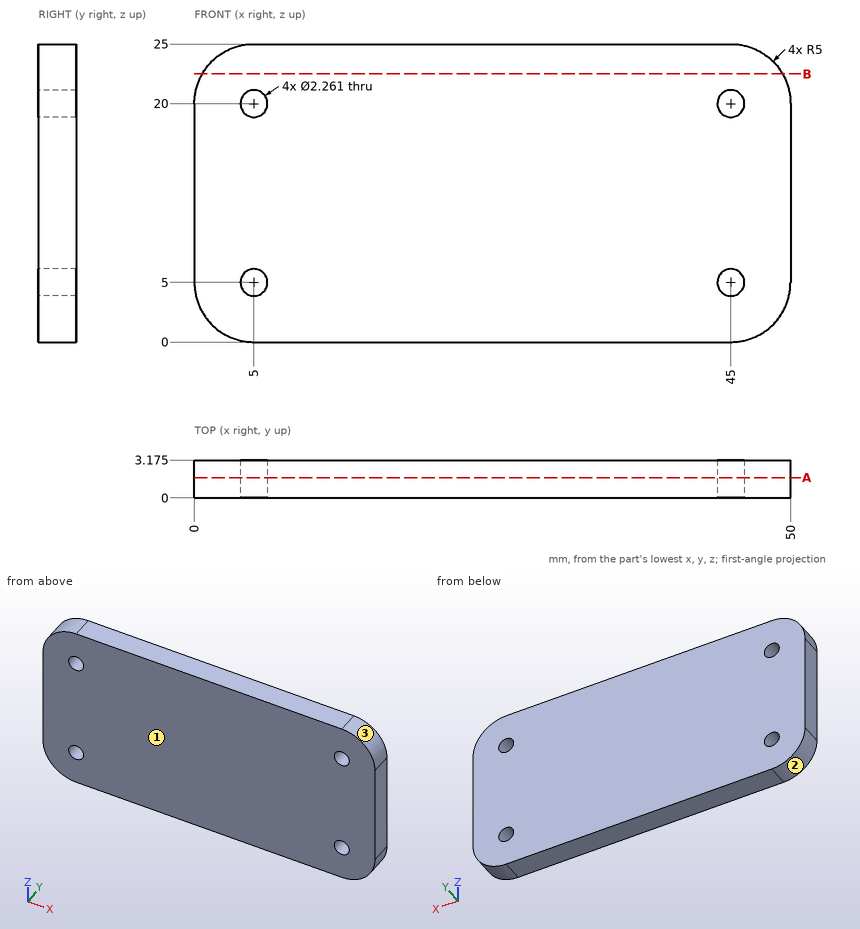
Source: three-view drawing plus pictorial views. Frame: mm from the lowest corner of the part. Coordinates: 2 decimals unless noted, no trailing zeros. Loops run counter-clockwise (first coordinate to the right, second up) from the corner with the lowest first, then second, coordinate; pieces in that order, holes last. Notation, with made-up numbers: (-38, 54) - (-17, 54) arc R28 ccw to (-17, 74) - close; hole circle Ø3 at (75.25, 64.5). An arc over 180 degrees is marked (long way). Answer in a Markdown table with one row per item. Add a question column.
Item 1: Section query B-B on z = 22.5. Return the cut outline in (x, y) (1 decimal).
Item 2: Contact query for a flat-ended pin moving along its axis: P1, Ø1.4, axis at x = 45, z = 20, coming from the +Y side. Output: stop coordinate, or through.
Item 3: Mould query, pull axis X, two halves, no side actions, for the marked faces 1, 2 and 3. Classes: released by +X, released by -X, zero draft, split by the parting line, or undercut.
Item 4: Section query A-A on y = 1.7. Return the cut outline in (x, z).
Item 5: Line query: line 1 along X through (y, z) = (2.15, 5); line 2 along Z through (x, y) = (5.5, 0.3) (1 decimal); line 3 along X through (y, z) = (0.85, 19) (1 decimal). Output: solid intervals per line, ascending. Write a range as [from, to].
Recorded:
| question | item | result |
|---|---|---|
| 1 | outline | (0.7, 0) - (49.3, 0) - (49.3, 3.2) - (0.7, 3.2) - close |
| 2 | P1 | through |
| 3 | face 1 | zero draft |
| 3 | face 2 | released by -X |
| 3 | face 3 | released by +X |
| 4 | outline | (0, 5) arc R5 ccw to (5, 0) - (45, 0) arc R5 ccw to (50, 5) - (50, 20) arc R5 ccw to (45, 25) - (5, 25) arc R5 ccw to (0, 20) - close; hole circle Ø2.26 at (5, 5); hole circle Ø2.26 at (5, 20); hole circle Ø2.26 at (45, 5); hole circle Ø2.26 at (45, 20) |
| 5 | line 1 | [0, 3.87], [6.13, 43.87], [46.13, 50] |
| 5 | line 2 | [0, 4], [6, 19], [21, 25] |
| 5 | line 3 | [0, 4.5], [5.5, 44.5], [45.5, 50] |
